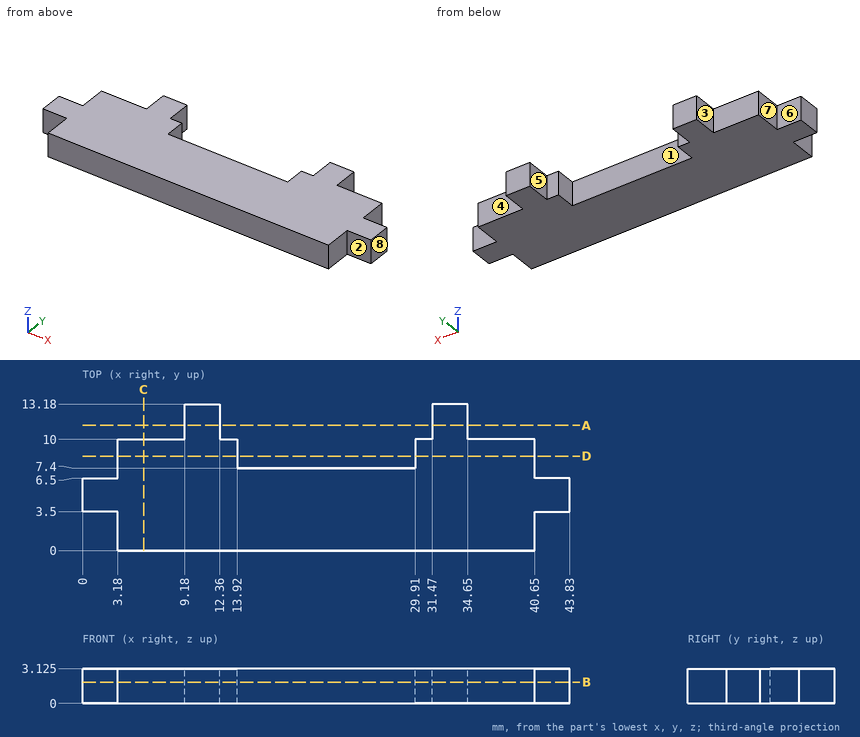
Source: three-view drawing plus pictorial views. Frame: mm from the lowest corner of the part. A direction names the side the tool comes from. Round coordinates to 2 decimals unless told otherwise and drop trailing zeros. Order: outer loops, then holes, each group sorted by start corner. A loop starts at its lowest first (then second) coordinate and runs counter-clockwise, first axis right, second up. Notation, with made-up numbers: (65, -14.5) -> (115, -14.5) arc R19 cw to (115, -3.5) -> close; hole circle Ø9 at (19, 82.5). An arc over 180 degrees is marked (long way). Use one line per item in the form item = value. Start each with the question number.
1. Reachability of the marked faces 1, 2, 3 and 4 from +Z, -Z, +X, -X, +Y, -Y: full face, straight path, thin tool, end or side. Return the list, or none.
2. Cut plane A-A (y = 11.25). Return the cut outline in (x, z) (3 decimals), then the cut area to 3 significant figures.
3. Cut plane C-C (x = 5.5). Return the cut outline in (y, z) (3 decimals), then the cut area to 4 significant figures.
4. Cut plane D-D (y = 8.5). Return the cut outline in (x, z) (3 decimals).
5. Pin query (flat end, axial travel): pin 1 Ø1.6 at (y, z) = (11, 1) entering from -X; pin 2 Ø1 at (y, z) = (10, 1.5) entering from -X; pin 3 Ø1.2 at (x, z) = (13.5, 1.5) entering from +Y. Return the tip coordinate at first contact, or that it passes through.
6. Draft query along X for the marked faces 5, 6, 7 and 8. Return one class per face: pulls with the +X half, pulls with the -X half, needs draft (parallel to the pull), parting line crosses it, or undercut.
7. Line query: probe 1 along X at (y, z) = (9, 0.5); probe 2 along Y at (x, z) = (26.5, 2.7); probe 3 along X at (y, z) = (7, 1.7). Output: solid intervals per line, ascending.
8. Cut plane B-B (z = 1.9). Return the cut outline in (x, y).
Solution:
q1.face_1 = +Z, -Z, +Y
q1.face_2 = +Z, -Z, +X, -Y
q1.face_3 = +Z, -Z, -X, +Y
q1.face_4 = +Z, -Z, +X, +Y
q2.outline = (9.18, 0) -> (12.36, 0) -> (12.36, 3.125) -> (9.18, 3.125) -> close; (31.47, 0) -> (34.65, 0) -> (34.65, 3.125) -> (31.47, 3.125) -> close
q2.area = 19.9 mm^2
q3.outline = (0, 0) -> (10, 0) -> (10, 3.125) -> (0, 3.125) -> close
q3.area = 31.25 mm^2
q4.outline = (3.18, 0) -> (13.92, 0) -> (13.92, 3.125) -> (3.18, 3.125) -> close; (29.91, 0) -> (40.65, 0) -> (40.65, 3.125) -> (29.91, 3.125) -> close
q5.pin_1 = 9.18
q5.pin_2 = 3.18
q5.pin_3 = 10
q6.face_5 = undercut
q6.face_6 = needs draft
q6.face_7 = pulls with the -X half
q6.face_8 = pulls with the +X half
q7.probe_1 = 3.18 to 13.92, 29.91 to 40.65
q7.probe_2 = 0 to 7.4
q7.probe_3 = 3.18 to 40.65
q8.outline = (0, 3.5) -> (3.18, 3.5) -> (3.18, 0) -> (40.65, 0) -> (40.65, 3.5) -> (43.83, 3.5) -> (43.83, 6.5) -> (40.65, 6.5) -> (40.65, 10) -> (34.65, 10) -> (34.65, 13.18) -> (31.47, 13.18) -> (31.47, 10) -> (29.91, 10) -> (29.91, 7.4) -> (13.92, 7.4) -> (13.92, 10) -> (12.36, 10) -> (12.36, 13.18) -> (9.18, 13.18) -> (9.18, 10) -> (3.18, 10) -> (3.18, 6.5) -> (0, 6.5) -> close
